Autodesk Inventor part; units mm, degrees
ref_plane "YZ Plane" through (0, 0, 0) normal (1, 0, 0) x (0, 1, 0)
ref_plane "XZ Plane" through (0, 0, 0) normal (0, 1, 0) x (-1, 0, 0)
ref_plane "XY Plane" through (0, 0, 0) normal (0, 0, 1) x (1, 0, 0)
sketch "Main Sketch" plane through (0, 0, 0) normal (0, 1, 0) x (-1, 0, 0)
  line L0 (0, 0) -> (-61, 0)
  line L1 (-61, 0) -> (-61, -52)
  line L2 (-61, -52) -> (0, -52)
  line L3 (0, -52) -> (0, 0)
  circle A0 centre (-7.5, -7.5) radius 1.5
  circle A1 centre (-7.5, -16.5) radius 1.5
  circle A2 centre (-7.5, -25.5) radius 1.5
  circle A3 centre (-19.5, -6.5) radius 1.5
  circle A4 centre (-45.5, -6.5) radius 1.5
  circle A5 centre (-19.5, -32.5) radius 1.5
  circle A6 centre (-45.5, -32.5) radius 1.5
  circle A7 centre (-7.5, -44.5) radius 1.5
  circle A8 centre (-45.5, -44.5) radius 1.5
  circle A9 centre (-57, -20.5) radius 1.5
  circle A10 centre (-32.5, -19.5) radius 11.1125
  dimension "d126" = 61
  dimension "d127" = 52
  dimension "d128" = 3
  dimension "d129" = 7.5
  dimension "d130" = 25.5
  dimension "d131" = 16.5
  dimension "d132" = 7.5
  dimension "d133" = 3
  dimension "d134" = 6.5
  dimension "d135" = 19.5
  dimension "d137" = 45.5
  dimension "d138" = 32.5
  dimension "d139" = 44.5
  dimension "d159" = 57
  dimension "d160" = 20.5
  dimension "d175" = 22.225
  dimension "d176" = 32.5
  dimension "d177" = 19.5
extrude "Extrusion10" add sketch "Main Sketch" against normal blind 7.5 contours L3 L2 L1 L0 | A0 | A1 | A2 | A3 | A4 | A5 | A6 | A7 | A8 | A9 | A10
hole "Hole14" at (19.5, 0, -32.5) at (45.5, 0, -32.5) at (45.5, 0, -6.5) at (19.5, 0, -6.5) direction (0, -1, 0) diameter 3.4036 end through all
hole "Frame Mounting Holes" at (7.5, 0, -16.5) at (7.5, 0, -44.5) at (45.5, 0, -44.5) direction (0, -1, 0) diameter 3.4036 end through all counterbore diameter 6.5024 counterbore depth 2.5
hole "Hole16" at (57, 0, -20.5) direction (0, -1, 0) diameter 2.459 end through all
hole "Pin Mounting Holes" at (7.5, 0, -25.5) at (7.5, 0, -7.5) direction (0, -1, 0) diameter 3.4036 depth 5 tip angle 118
hole "Hole18" at (32.5, 0, -19.5) direction (0, -1, 0) diameter 22.225 end through all
sketch "Sketch15" plane through (0, -7.5, 0) normal (0, -1, 0) x (1, 0, 0)
  circle A0 centre (32.5, -19.5) radius 11.1125
  circle A1 centre (57, -20.5) radius 1.2295
  circle A2 centre (7.5, -16.5) radius 1.7018
  circle A3 centre (19.5, -6.5) radius 1.7018
  circle A4 centre (45.5, -6.5) radius 1.7018
  circle A5 centre (45.5, -32.5) radius 1.7018
  circle A6 centre (19.5, -32.5) radius 1.7018
  line L0 (61, -52) -> (61, 0)
  line L1 (61, 0) -> (0, 0)
  line L2 (0, 0) -> (0, -52)
  line L3 (0, -52) -> (61, -52)
  line L4 (14.8, -1.8) -> (50.2, -1.8)
  line L5 (50.2, -1.8) -> (50.2, -37.2)
  line L6 (50.2, -37.2) -> (14.8, -37.2)
  line L7 (14.8, -37.2) -> (14.8, -1.8)
  dimension "d185" = 14.8
  dimension "d186" = 1.8
  dimension "d187" = 35.4
  dimension "d188" = 35.4
extrude "Extrusion11" cut sketch "Sketch15" against normal blind 5 contours L4 L5 L6 L7
fillet "Fillet1" radius 3.175 4 edges at (14.8, -5, -1.8) (50.2, -5, -1.8) (50.2, -5, -37.2) (14.8, -5, -37.2)
fillet "Fillet2" radius 6.35 3 edges at (61, -3.75, 0) (61, -3.75, -52) (0, -3.75, -52)
equation "\"d131\" = 0.5 * d130 + 0.5 * d129"
properties part number "A Drive Frame Lower" material "Aluminum 6061"
Work out the finished part from the listing and answer in its coordinate system (mm). A direction names the side the tool comes from. Coordinates: 2 decimals unless noted, no trailing zeros. Write each loop counter-clockwise with the first axis right and the second up, starting at its lowest first coordinate (ties: lowest second). Pieces come first, ordered by that corner, then holes. Notation, with made-up numbers: (15, -13.5) - (56, -13.5) arc R25 ccw to (56, 0.5) - close; hole circle Ø7 at (19.5, 15). An arc over 180 degrees is marked (long way). One line per question, with ' | ' between items.
1) For faces 1 (the face through (6.35, -2.535, -8.754)), 2 (the face through (31, 0, -31)), 3 (the face through (15.71, -4.96, -2.75)), determine the directions among +Z, -Z, +X, -X, +Y, -Y from which every point of the face is accessible in a straight line to the end or side of a thin tool.
Checks:
face 1: +Y | face 2: +Z, -Z, +X, -X, +Y | face 3: -Y
2) Find section C-C, the plane y = -0.75. Give the number of separate pieces and of enclosed holes in the cut face, and give its area (3 significant figures).
Checks:
separate pieces: 1 | enclosed holes: 11 | area: 2,600 mm2
3) Find section A-A, the plane x = 19.5. Determine the outline of the cut face in (y, z), and give its area (3 significant figures).
Checks:
outline: (-7.5, -52) - (0, -52) - (0, -34.2) - (-2.5, -34.2) - (-2.5, -37.2) - (-7.5, -37.2) - close; (-7.5, -1.8) - (-2.5, -1.8) - (-2.5, -4.8) - (0, -4.8) - (0, 0) - (-7.5, 0) - close; (-2.5, -30.8) - (0, -30.8) - (0, -8.2) - (-2.5, -8.2) - close | area: 196 mm2
4) Find section D-D, the plane x = 45.5. Determine the outline of the cut face in (y, z).
Checks:
outline: (-7.5, -52) - (0, -52) - (0, -47.75) - (-2.5, -47.75) - (-2.5, -46.2) - (-7.5, -46.2) - close; (-7.5, -42.8) - (-2.5, -42.8) - (-2.5, -41.25) - (0, -41.25) - (0, -34.2) - (-2.5, -34.2) - (-2.5, -37.2) - (-7.5, -37.2) - close; (-7.5, -1.8) - (-2.5, -1.8) - (-2.5, -4.8) - (0, -4.8) - (0, 0) - (-7.5, 0) - close; (-2.5, -30.8) - (0, -30.8) - (0, -8.2) - (-2.5, -8.2) - close
5) Flat-ended cylindrical pins translate along their axes: P1, Ø2.5, axis at x = 45.5, z = -44.5, coming from the -Y side; P2, Ø12, axis at x = 30.5, z = -40.5, coming from the +Y side; P3, Ø4.5, axis at x = 19.5, z = -6.5, coming from the -Y side; P4, Ø3.5, axis at x = 46, z = -44.5, coming from the +Y side. Find the tip coordinate at first contact, or state that the pin passes through.
Checks:
P1: through | P2: y = 0 | P3: y = -2.5 | P4: y = -2.5
6) Find section B-B, the plane z = -32.5. Determine the outline of the cut face in (x, y), and give its area (3 significant figures).
Checks:
outline: (0, -7.5) - (14.8, -7.5) - (14.8, -2.5) - (17.8, -2.5) - (17.8, 0) - (0, 0) - close; (21.2, -2.5) - (43.8, -2.5) - (43.8, 0) - (21.2, 0) - close; (47.2, -2.5) - (50.2, -2.5) - (50.2, -7.5) - (61, -7.5) - (61, 0) - (47.2, 0) - close | area: 263 mm2
7) The mould has two halves that part along X. Classify faces 4 (the face through (0, -4, -23)), 5 (the face through (59.19, -3.8, -1.91)), 6 (the face through (31, -4, -52)), 7 (the face through (32, -5, -1.8)): +X half, -X half, draft (parallel to the pull), parting line (faces both ways), or undercut.
Checks:
face 4: -X half | face 5: +X half | face 6: draft | face 7: undercut
8) Consider probe 1 along Z at (x, y) = (45.5, -1.7); probe 2 along X at (y, z) = (-3.95, -16.5); probe 3 along Z at (x, y) = (19.5, -2). Determine where each line is inside the solid, lowest interval first. Write a range as [from, to].
Checks:
probe 1: [-52, -47.75], [-41.25, -34.2], [-30.8, -8.2], [-4.8, 0] | probe 2: [0, 5.8], [9.2, 14.8], [50.2, 61] | probe 3: [-52, -34.2], [-30.8, -8.2], [-4.8, 0]
